Geometry: final body of the model. Coordinates: model frame, mm. Face numbers are marked on the shaded views. A direction names the side the tool comes from. Give positions to 0.01 mm unless a question says otherwise; leave off trailing zeros. Order: outer loops, then holes, each group sorted by start corner. A loop starts at its lowest first (then second) coordinate and runs counter-clockwise, first axis right, second up. Notation, with made-up numbers: (-31.5, 33.25) -> (8.5, 33.25) arc R24 cw to (8.5, 44.25) -> close; hole circle Ø3 at (52.5, 72.5). An arc over 180 degrees is marked (long way). Write item = value, one per line.
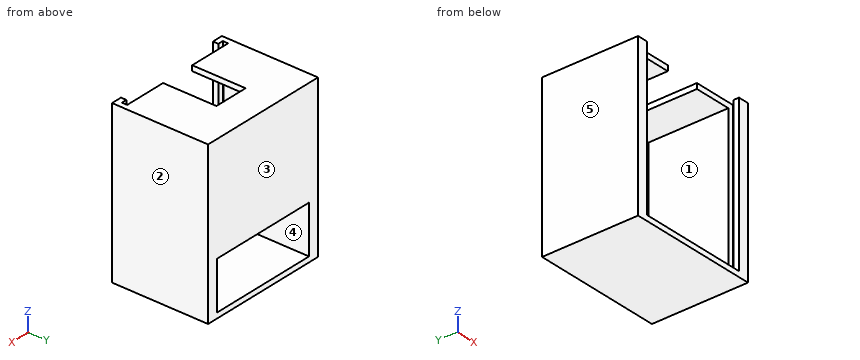
```python
from build123d import *

# Parameters (mm, degrees)
ESQUISSE1_W                  = 24.5
ESQUISSE1_H                  = 18
BOSS_EXTRU_3_DEPTH           = 30
ENL_V_MAT_EXTRU_1_DEPTH      = 43.711239739
ENL_V_MAT_EXTRU_1_DEPTH_BACK = 29
ENL_V_MAT_EXTRU_2_DEPTH      = 1
ESQUISSE6_W                  = 29
ESQUISSE6_H                  = 1
ENL_V_MAT_EXTRU_3_DEPTH      = 1
ESQUISSE7_W                  = 20.5
ESQUISSE7_H                  = 15
BOSS_EXTRU_4_DEPTH           = 1
ESQUISSE8_W                  = 6.5
ESQUISSE8_H                  = 10
ENL_V_MAT_EXTRU_4_DEPTH      = 1
ESQUISSE10_W                 = 20.5
ESQUISSE10_H                 = 9
ENL_V_MAT_EXTRU_5_DEPTH      = 43.299527184


with BuildPart() as part:
    # Esquisse1 → Boss.-Extru.3 (new body)
    with BuildSketch(Plane.XY):
        with Locations((12.25, 9)):
            Rectangle(ESQUISSE1_W, ESQUISSE1_H)
    extrude(amount=BOSS_EXTRU_3_DEPTH)

    # Esquisse4 → Enlèv. mat.-Extru.1 (cut, two sides: drawn at the far end of the back side and taken through both)
    with BuildSketch(Plane.XY.offset(30).offset(-ENL_V_MAT_EXTRU_1_DEPTH_BACK)):
        Polygon((22.5, -67.628118137), (22.5, 0), (22.5, 17), (2, 17), (2, 0), (2, -67.628118137), (2, -202.884354411), (22.5, -202.884354411), align=None)
    extrude(amount=ENL_V_MAT_EXTRU_1_DEPTH + ENL_V_MAT_EXTRU_1_DEPTH_BACK, mode=Mode.SUBTRACT)

    # Esquisse5 → Enlèv. mat.-Extru.2 (cut)
    with BuildSketch(Plane(origin=(2, 0, 0), x_dir=(0, 0, -1), z_dir=(1, 0, 0))):
        Polygon((-1, 1), (-30, 1), (-30, 2), (-2, 2), (-1, 2), align=None)
    extrude(amount=-ENL_V_MAT_EXTRU_2_DEPTH, mode=Mode.SUBTRACT)

    # Esquisse6 → Enlèv. mat.-Extru.3 (cut)
    with BuildSketch(Plane.ZY.offset(-22.5)):
        with Locations((15.5, 1.5)):
            Rectangle(ESQUISSE6_W, ESQUISSE6_H)
    extrude(amount=-ENL_V_MAT_EXTRU_3_DEPTH, mode=Mode.SUBTRACT)

    # Esquisse7 → Boss.-Extru.4 (add)
    with BuildSketch(Plane.XY.offset(30)):
        with Locations((12.25, 9.5)):
            Rectangle(ESQUISSE7_W, ESQUISSE7_H)
    extrude(amount=-BOSS_EXTRU_4_DEPTH)

    # Esquisse8 → Enlèv. mat.-Extru.4 (cut)
    with BuildSketch(Plane.XY.offset(30)):
        with Locations((12.25, 7)):
            Rectangle(ESQUISSE8_W, ESQUISSE8_H)
    extrude(amount=-ENL_V_MAT_EXTRU_4_DEPTH, mode=Mode.SUBTRACT)

    # Esquisse10 → Enlèv. mat.-Extru.5 (cut, through all)
    with BuildSketch(Plane(origin=(0, 17, 0), x_dir=(-1, 0, 0), z_dir=(0, -1, 0))):
        with Locations((-12.25, -5.5)):
            Rectangle(ESQUISSE10_W, ESQUISSE10_H)
    extrude(amount=-ENL_V_MAT_EXTRU_5_DEPTH, mode=Mode.SUBTRACT)


solid = part.part
```
1) First-contact query: P1, Ø1.5, axis at x = 17, z = 26, coming from the -Y side. Flat tip, straight axial feed; report the tip coordinate or a pass-through.
Check sheet entries:
P1 = 17
2) Mould query, pull axis X, two halves, no side actions, for the marked faces 3, 4 and 5. Classes: +X half, -X half, draft (parallel to the pull), parting line (faces both ways), or undercut.
Check sheet entries:
face_3 = draft
face_4 = undercut
face_5 = -X half
3) Line query: line 1 (Z direction, x = 3.5, y = 7.5); line 2 (X direction, y = 10.75, z = 9.25); line 3 (Z direction, x = 9.25, y = 0.5). Output: solid intervals per line, ascending. Write a range as from..to.
Check sheet entries:
line_1 = 0..1, 29..30
line_2 = 0..2, 22.5..24.5
line_3 = 0..1
4) Reachability of the marked faces 1 and 2 from +Z, -Z, +X, -X, +Y, -Y: full face, straight path, thin tool, end or side. Return the list, or none.
Check sheet entries:
face_1 = -Y
face_2 = +Z, -Z, +X, +Y, -Y
5) Section query B-B (x = 7). Output: boundary loops of the cut face in (y, z).
Check sheet entries:
outline = (0, 0) -> (18, 0) -> (18, 1) -> (0, 1) -> close; (2, 29) -> (17, 29) -> (17, 10) -> (18, 10) -> (18, 30) -> (2, 30) -> close
6) Section query D-D (y = 3). Output: boundary loops of the cut face in (x, z), plus the area to 4 significant figures.
Check sheet entries:
outline = (0, 0) -> (24.5, 0) -> (24.5, 30) -> (15.5, 30) -> (15.5, 29) -> (22.5, 29) -> (22.5, 1) -> (2, 1) -> (2, 29) -> (9, 29) -> (9, 30) -> (0, 30) -> close
area = 154.5 mm²
7) Section query A-A (z = 3). Output: boundary loops of the cut face in (x, y), plus the area to 3 significant figures.
Check sheet entries:
outline = (0, 0) -> (2, 0) -> (2, 1) -> (1, 1) -> (1, 2) -> (2, 2) -> (2, 18) -> (0, 18) -> close; (22.5, 0) -> (24.5, 0) -> (24.5, 18) -> (22.5, 18) -> (22.5, 2) -> (23.5, 2) -> (23.5, 1) -> (22.5, 1) -> close
area = 70.0 mm²
8) Section query C-C (y = 16.25). Output: boundary loops of the cut face in (x, z), plus the area to 3 significant figures.
Check sheet entries:
outline = (0, 0) -> (24.5, 0) -> (24.5, 30) -> (0, 30) -> close; hole (2, 1) -> (22.5, 1) -> (22.5, 29) -> (2, 29) -> close
area = 161 mm²
